Geometry: final body of the model. Coordinates: model frame, mm. Face numbers are marked on the shaded views. A direction names the side the tool comes from. Give positions to 0.01 mm unless a question says otherwise; leave off trailing zeros. Write each loop counter-clockwise with the first axis right and the second up, starting at its lowest first coordinate (ties: lowest second). Pieces come first, ordered by that corner, then holes.
Q1. Cut plane A-A on x = -30. Return the cut outline in (y, z).
Q2. Pin query (flat end, axial travel): pin 1 (17.5 mm diameter, centred on x = 53.54, z = -47.25, fed in from +Y); pin 2 (25 mm diameter, centred on x = -1, y = 36.5, fed in from +Z); pin 3 (6 mm diameter, centred on y = 51, z = 6.5, fed in from -X). Return the tip coordinate at first contact, or that it passes through.
Q3. Draft query along Z for the marked faces 1, 2 and 3. Return one class per face: pulls with the +Z half, pulls with the -Z half, needs draft (parallel to the pull), parting line crosses it, or undercut.
Q4. Cut plane D-D on y = 18. Return the cut outline in (x, z), plus the area to 3 significant figures.
Q5. Cut plane B-B on z = -10.5. Return the cut outline in (x, y), plus the area to 3 significant figures.
Q6. Reachability of the marked faces 4 and 5 from +Z, -Z, +X, -X, +Y, -Y: full face, straight path, thin tool, end or side. Return the list, or none.
Q7. Line query: L1, parallel to X at y = 27, z = 21.5; L2, parallel to Z at x = -4, y = 47; L3, parallel to X at y = 7, z = -41.5. Output: solid intervals per line, ascending.
Q8. Cut plane C-C on x = 31. Return the cut outline in (y, z), plus the area to 3 significant figures.
```python
from build123d import *

# Parameters (mm, degrees)
SKETCH1_W                                    = 157
SKETCH1_H                                    = 160
BOSS_EXTRUDE1_DEPTH                          = 10
SKETCH2_W                                    = 61
SKETCH2_H                                    = 64
CUT_EXTRUDE1_DEPTH                           = 10
CBORE_SLOT_FOR_M12_HEX_HEAD_BOLT1_AT_2_COUNT = 2
CBORE_SLOT_FOR_M12_HEX_HEAD_BOLT1_AT_2_PITCH = 111.420621054
CBORE_SLOT_FOR_M12_HEX_HEAD_BOLT1_AT_3_COUNT = 2
CBORE_SLOT_FOR_M12_HEX_HEAD_BOLT1_AT_3_PITCH = 160.357529077
CBORE_SLOT_FOR_M12_HEX_HEAD_BOLT1_AT_4_COUNT = 2
CBORE_SLOT_FOR_M12_HEX_HEAD_BOLT1_AT_4_PITCH = 115.325549362
SKETCH7_W                                    = 87
SKETCH7_H                                    = 90
SKETCH7_W_2                                  = 77
SKETCH7_H_2                                  = 80
EXTRUDE_THIN1_DEPTH                          = 50


with BuildPart() as part:
    # Sketch1 → Boss-Extrude1 (new body)
    with BuildSketch(Plane(origin=(0, 0, 0), x_dir=(1, 0, 0), z_dir=(0, 1, 0))):
        with Locations((-1.646853147, -10.283216783)):
            Rectangle(SKETCH1_W, SKETCH1_H)
    extrude(amount=BOSS_EXTRUDE1_DEPTH)

    # Sketch2 → Cut-Extrude1 (cut)
    with BuildSketch(Plane(origin=(0, 10, 0), x_dir=(1, 0, 0), z_dir=(0, 1, 0))):
        with Locations((-1.646853147, -10.283216783)):
            Rectangle(SKETCH2_W, SKETCH2_H)
    extrude(amount=-CUT_EXTRUDE1_DEPTH, mode=Mode.SUBTRACT)

    # Sketch4 → CBORE SLOT for M12 Hex Head Bolt1 (revolve, cut)
    with BuildSketch(Plane(origin=(-57.877820781, 10, -47.249393621), x_dir=(0, 0, 1), z_dir=(1, 0, 0))):
        Polygon((0, 0), (0, 22.055809178), (6.75, 18), (6.75, 7.95), (11.89, 7.95), (11.89, 1.135), (13.025, 0), align=None)
    cbore_slot_for_m12_hex_head_bolt1 = revolve(axis=Axis((-57.877820781, 16.35, -47.249393621), (0, -1, 0)), mode=Mode.SUBTRACT)

    # CBORE SLOT for M12 Hex Head Bolt1 at 2: CBORE SLOT for M12 Hex Head Bolt1 ×2
    with Locations(*[(i * CBORE_SLOT_FOR_M12_HEX_HEAD_BOLT1_AT_2_PITCH, 0, 0) for i in range(1, CBORE_SLOT_FOR_M12_HEX_HEAD_BOLT1_AT_2_COUNT)]):
        add(cbore_slot_for_m12_hex_head_bolt1, mode=Mode.SUBTRACT)

    # CBORE SLOT for M12 Hex Head Bolt1 at 3: CBORE SLOT for M12 Hex Head Bolt1 ×2
    with Locations(*[Vector(0.6948262529067781, 0, 0.7191776402750062) * (i * CBORE_SLOT_FOR_M12_HEX_HEAD_BOLT1_AT_3_PITCH) for i in range(1, CBORE_SLOT_FOR_M12_HEX_HEAD_BOLT1_AT_3_COUNT)]):
        add(cbore_slot_for_m12_hex_head_bolt1, mode=Mode.SUBTRACT)

    # CBORE SLOT for M12 Hex Head Bolt1 at 4: CBORE SLOT for M12 Hex Head Bolt1 ×2
    with Locations(*[(0, 0, i * CBORE_SLOT_FOR_M12_HEX_HEAD_BOLT1_AT_4_PITCH) for i in range(1, CBORE_SLOT_FOR_M12_HEX_HEAD_BOLT1_AT_4_COUNT)]):
        add(cbore_slot_for_m12_hex_head_bolt1, mode=Mode.SUBTRACT)

    # Sketch7 → Extrude-Thin1 (add)
    with BuildSketch(Plane(origin=(0, 10, 0), x_dir=(1, 0, 0), z_dir=(0, 1, 0))):
        with Locations((-1.646853147, -10.283216783)):
            Rectangle(SKETCH7_W, SKETCH7_H)
        with Locations((-1.646853147, -10.283216783)):
            Rectangle(SKETCH7_W_2, SKETCH7_H_2, mode=Mode.SUBTRACT)
    extrude(amount=EXTRUDE_THIN1_DEPTH)


solid = part.part
```
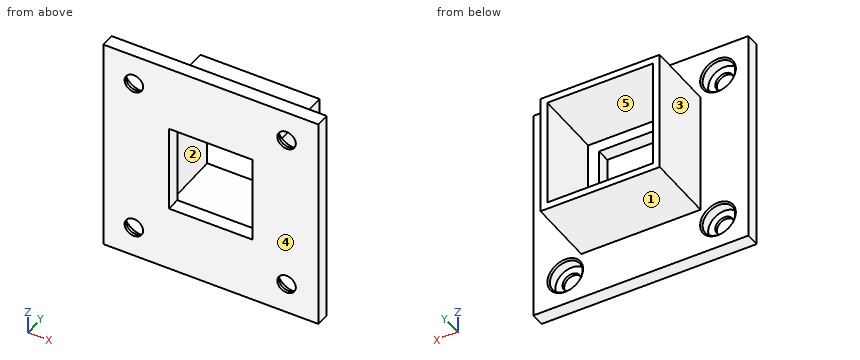
Data:
1. outline: (0, -69.72) - (10, -69.72) - (10, -34.72) - (60, -34.72) - (60, -29.72) - (10, -29.72) - (10, -21.72) - (0, -21.72) - close; (0, 42.28) - (10, 42.28) - (10, 50.28) - (60, 50.28) - (60, 55.28) - (10, 55.28) - (10, 90.28) - (0, 90.28) - close
2. pin 1: stops at y = 2.05
2. pin 2: stops at z = 55.28
2. pin 3: stops at x = -45.15
3. face 1: pulls with the -Z half
3. face 2: undercut
3. face 3: needs draft
4. outline: (-45.15, -34.72) - (41.85, -34.72) - (41.85, 55.28) - (-45.15, 55.28) - close; hole (-40.15, -29.72) - (36.85, -29.72) - (36.85, 50.28) - (-40.15, 50.28) - close
4. area: 1,670 mm2
5. outline: (-80.15, 0) - (-32.15, 0) - (-32.15, 10) - (-40.15, 10) - (-40.15, 60) - (-45.15, 60) - (-45.15, 10) - (-80.15, 10) - close; (28.85, 0) - (76.85, 0) - (76.85, 10) - (41.85, 10) - (41.85, 60) - (36.85, 60) - (36.85, 10) - (28.85, 10) - close
5. area: 1,460 mm2
6. face 4: +Z, -Z, +X, -X, -Y
6. face 5: +Y
7. L1: x = -45.15 to -40.15, 36.85 to 41.85
7. L2: z = -34.72 to -29.72, 50.28 to 55.28
7. L3: x = -80.15 to -68.29, -47.47 to 43.14, 63.95 to 76.85
8. outline: (0, -69.72) - (10, -69.72) - (10, -34.72) - (60, -34.72) - (60, -29.72) - (10, -29.72) - (10, 50.28) - (60, 50.28) - (60, 55.28) - (10, 55.28) - (10, 90.28) - (0, 90.28) - close
8. area: 2,100 mm2
